Design review of the part built by this model. Coordinates are the model's own, in mm. Coordinates: 2 decimals unless noted, no trailing zeros. Write each loop counter-clockwise with the first axis right and the second up, starting at its lowest first coordinate (ties: lowest second). Pieces come first, ordered by that corner, then holes. Notation, with made-up numbers: (-40, 9.5) -> (-34, 9.5) arc R11 ccw to (-34, 29.5) -> close; hole circle Ø11 at (-39.5, -7.75). An arc over 180 degrees is marked (long way). Answer in a Markdown table with one row per item. Add a question column.
Item 1: Take a section at A-A, the plane y = 0.5. Write out the cut boundary in (x, z).
Item 2: Take a section at C-C, the plane x = -3. Write out the cut boundary in (y, z), and give its area (3 significant figures).
Item 3: Clearance check with flat-ended pins moving along their axes: P1, Ø1.5, axis at x = 33, z = 0.5, coming from the -Y side; P2, Ø0.9, axis at y = 13, z = -0.5, coming from the +X side. State where each tip first meets the part, or that it passes through.
Item 4: Take a section at D-D, the plane y = -14. Write out the cut boundary in (x, z), and give its area (3 significant figures).
Item 5: Take a section at B-B, the plane z = -0.7. Write out the cut boundary in (x, y).
Item 6: To check wall thickness, follow line 1 (Y direction, x = 17, z = -0.6); line 2 (X direction, y = 9.5, z = 0.5); line 3 (X direction, y = 13, z = -0.3). State the ranges of each line that lie inside material, in increasing order.
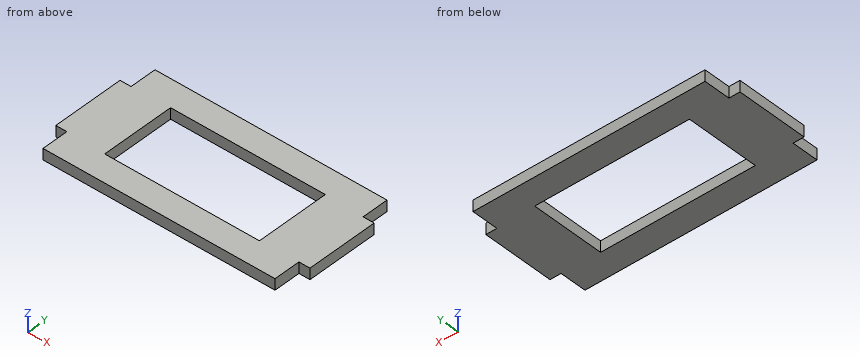
Autodesk Inventor part; units mm, degrees
ref_plane "YZ Plane" through (0, 0, 0) normal (1, 0, 0) x (0, 1, 0)
ref_plane "XZ Plane" through (0, 0, 0) normal (0, 1, 0) x (-1, 0, 0)
ref_plane "XY Plane" through (0, 0, 0) normal (0, 0, 1) x (1, 0, 0)
sketch "Sketch1" plane through (0, 0, 0) normal (0, 0, 1) x (1, 0, 0)
  line L0 (-34.5, 17) -> (34.5, 17)
  line L1 (34.5, 17) -> (34.5, -17)
  line L2 (34.5, -17) -> (-34.5, -17)
  line L3 (-34.5, -17) -> (-34.5, 17)
  line L4 (34.5, 9.75) -> (31.5, 9.75)
  line L5 (31.5, 9.75) -> (31.5, -9.75)
  line L6 (31.5, -9.75) -> (34.5, -9.75)
  line L7 (34.5, -9.75) -> (34.5, 9.75)
  line L8 (-21, 10) -> (21, 10)
  line L9 (21, 10) -> (21, -10)
  line L10 (21, -10) -> (-21, -10)
  line L11 (-21, -10) -> (-21, 10)
  line L12 (0, 31.4058) -> (0, -31.4058)
  line L13 (31.5, 17) -> (31.5, 9.75)
  line L14 (31.5, -9.75) -> (31.5, -17)
  line L15 (-34.5, 17) -> (-34.5, -17)
  line L16 (-34.5, 9.75) -> (-31.5, 9.75)
  line L17 (-31.5, 9.75) -> (-31.5, -9.75)
  line L18 (-31.5, -9.75) -> (-34.5, -9.75)
  line L19 (-31.5, 17) -> (-31.5, 9.75)
  line L20 (-31.5, -9.75) -> (-31.5, -17)
  point P0 (0, 0)
  point P1 (34.5, 0)
  point P2 (0, 17)
  point P3 (34.5, 0)
  point P4 (21, 0)
  point P5 (0, 10)
  point P6 (-31, 17)
  point P7 (-31, -17)
  point P8 (31.5, -17)
  point P9 (0, 0)
  dimension "d0" = 34
  dimension "d1" = 19.5
  dimension "d2" = 3
  dimension "d3" = 20
  dimension "d4" = 69
  dimension "d5" = 42
extrude "Extrusion1" add sketch "Sketch1" along normal mid plane 3 contours L0 L12 L8 L11 L10 L2 L20 L17 L19 | L16 L17 L18 L3 | L0 L13 L5 L14 L2 L12 L10 L9 L8 | L4 L1 L6 L5
properties part number "C"
Answers:
| question | item | result |
|---|---|---|
| 1 | outline | (-34.5, -1.5) -> (-21, -1.5) -> (-21, 1.5) -> (-34.5, 1.5) -> close; (21, -1.5) -> (34.5, -1.5) -> (34.5, 1.5) -> (21, 1.5) -> close |
| 2 | outline | (-17, -1.5) -> (-10, -1.5) -> (-10, 1.5) -> (-17, 1.5) -> close; (10, -1.5) -> (17, -1.5) -> (17, 1.5) -> (10, 1.5) -> close |
| 2 | area | 42.0 mm^2 |
| 3 | P1 | stops at y = -9.75 |
| 3 | P2 | stops at x = 31.5 |
| 4 | outline | (-31.5, -1.5) -> (31.5, -1.5) -> (31.5, 1.5) -> (-31.5, 1.5) -> close |
| 4 | area | 189 mm^2 |
| 5 | outline | (-34.5, -9.75) -> (-31.5, -9.75) -> (-31.5, -17) -> (31.5, -17) -> (31.5, -9.75) -> (34.5, -9.75) -> (34.5, 9.75) -> (31.5, 9.75) -> (31.5, 17) -> (-31.5, 17) -> (-31.5, 9.75) -> (-34.5, 9.75) -> close; hole (-21, -10) -> (21, -10) -> (21, 10) -> (-21, 10) -> close |
| 6 | line 1 | y = -17 to -10, 10 to 17 |
| 6 | line 2 | x = -34.5 to -21, 21 to 34.5 |
| 6 | line 3 | x = -31.5 to 31.5 |
